Work out the finished part from the listing and answer in its coordinate system (mm). A direction names the side the tool comes from. Round coordinates to 2 decimals unless told otherwise and drop trailing zeros. Order: outer loops, then holes, each group sorted by start corner. A loop starts at its lowest first (then second) coordinate and runs counter-clockwise, first axis right, second up. Notation, with made-up numbers: (-16.5, 56.25) - (-11.5, 56.25) arc R38 cw to (-11.5, 94.25) - close; hole circle Ø3 at (34, 60.25). An arc over 180 degrees is marked (long way). One line per question, with ' | ' between items. Start each with the question number.
from build123d import *

# Parameters (mm, degrees)
F0_R      = 114
F1_DEPTH  = 25
F2_R      = 57
F3_DEPTH  = 200
F4_R      = 114
F5_DEPTH  = 25
F6_R      = 60
F7_DEPTH  = 100
F8_W      = 15
F8_H      = 150
F9_DEPTH  = 25
F10_R     = 9.5
F11_DEPTH = 30
F12_R     = 9.5
F13_DEPTH = 30
F14_R     = 51
F15_DEPTH = 1000


with BuildPart() as f1:
    # F0 (on Front) → F1 (new body)
    with BuildSketch(Plane.XZ):
        Circle(F0_R)
    extrude(amount=F1_DEPTH)

    # F2 (on face) → F3 (join)
    with BuildSketch(Plane.XZ.offset(25)):
        Circle(F2_R)
    extrude(amount=F3_DEPTH)

    # F4 (on face) → F5 (join)
    with BuildSketch(Plane.XZ.offset(225)):
        Circle(F4_R)
    extrude(amount=F5_DEPTH)

    # F6 (on Top) → F7 (join, symmetric)
    with BuildSketch(Plane.XY):
        with Locations((0, -125)):
            Circle(F6_R)
    extrude(amount=F7_DEPTH, both=True)

    # F8 (on face) → F9 (join)
    with BuildSketch(Plane.XY.offset(100)):
        with Locations((-0.883462, -205)):
            Rectangle(F8_W, F8_H)
    extrude(amount=F9_DEPTH)

    # F10 (on face) → F11 (cut)
    with BuildSketch(Plane.XZ.offset(250)):
        with Locations((0, 95)):
            Circle(F10_R)
        with Locations((-67.175144, 67.175144)):
            Circle(F10_R)
        with Locations((-95, 0)):
            Circle(F10_R)
        with Locations((-67.175144, -67.175144)):
            Circle(F10_R)
        with Locations((0, -95)):
            Circle(F10_R)
        with Locations((67.175144, -67.175144)):
            Circle(F10_R)
        with Locations((95, 0)):
            Circle(F10_R)
        with Locations((67.175144, 67.175144)):
            Circle(F10_R)
    extrude(amount=-F11_DEPTH, mode=Mode.SUBTRACT)

    # F12 (on face) → F13 (cut)
    with BuildSketch(Plane(origin=(0, 0, 0), x_dir=(-1, 0, 0), z_dir=(0, 1, 0))):
        with Locations((0, 95)):
            Circle(F12_R)
        with Locations((-67.175144, 67.175144)):
            Circle(F12_R)
        with Locations((-95, 0)):
            Circle(F12_R)
        with Locations((-67.175144, -67.175144)):
            Circle(F12_R)
        with Locations((0, -95)):
            Circle(F12_R)
        with Locations((67.175144, -67.175144)):
            Circle(F12_R)
        with Locations((95, 0)):
            Circle(F12_R)
        with Locations((67.175144, 67.175144)):
            Circle(F12_R)
    extrude(amount=-F13_DEPTH, mode=Mode.SUBTRACT)

    # F14 (on face) → F15 (cut)
    with BuildSketch(Plane(origin=(0, 0, 0), x_dir=(-1, 0, 0), z_dir=(0, 1, 0))):
        Circle(F14_R)
    extrude(amount=-F15_DEPTH, mode=Mode.SUBTRACT)


solid = f1.part
1) Straight lines are drawn through the part: line 1 (Y direction, x = 2, z = 76.5); line 2 (Z direction, x = 0, y = -16.5); line 3 (Z direction, x = 0, y = -234.75). For each, find the intervals that lie inside material, in ascending order.
2) Section D-D on x = 0 is taken. Give the number of separate pieces and of enclosed holes in the cut face, and give its area (3 significant figures).
3) Section B-B on x = -95 is taken. Give the vertices of the cut face in (y, z), and give its area (3 significant figures).
4) For faces 4 (the flat face through (-1, -265, 100)), 5 (the cylindrical face through (58.114, -12.325, -64.322)), 6 (the cylindrical face through (57.23, -106.98, 1.4)), determine the directions among +Z, -Z, +X, -X, +Y, -Y from which every point of the face is accessible in a straight line to the end or side of a thin tool.
5) Determine the mould class of faces 1 (the flat face through (-1, -280, 112)), 2 (the cylindrical face through (-104.061, -12.325, 2.854)), 3 (the cylindrical face through (-12.356, -192.828, -55.645)) for opening direction Y: released by +Y, released by -Y, zero draft, split by the parting line, or undercut.
6) Flat-ended cylindrical pins translate along their axes: pin 1 (8 mm diameter, centred on y = -168.5, z = -68.5, fed in from +X); pin 2 (12 mm diameter, centred on x = -4, y = -210.5, fed in from -Z); pin 3 (10 mm diameter, centred on x = 16.5, y = -129, fed in from -Z); pin 4 (11.5 mm diameter, centred on x = 67.18, z = -67.18, fed in from +Y). Find the tip coordinate at first contact, or state that the pin passes through.
7) Section A-A on y = -125 is taken. Give the vertices of the cut face in (x, z).
8) Section C-C on z = -95 is taken. Give the vertices of the cut face in (x, y).
Recorded:
1) line 1: y = -250 to -225, -184.97 to -65.03, -25 to 0 | line 2: z = -114 to -104.5, -85.5 to -51, 51 to 85.5, 104.5 to 114 | line 3: z = -114 to -104.5, -85.5 to -51, 51 to 85.5, 104.5 to 125
2) separate pieces: 5 | enclosed holes: 0 | area: 20,500 mm²
3) outline: (-250, -63.02) - (-225, -63.02) - (-225, -9.5) - (-250, -9.5) - close; (-250, 9.5) - (-225, 9.5) - (-225, 63.02) - (-250, 63.02) - close; (-25, -63.02) - (0, -63.02) - (0, -9.5) - (-25, -9.5) - close; (-25, 9.5) - (0, 9.5) - (0, 63.02) - (-25, 63.02) - close | area: 5,350 mm²
4) face 4: -Z, +X, -X, -Y | face 5: +Y | face 6: none
5) face 1: released by -Y | face 2: zero draft | face 3: undercut
6) pin 1: stops at x = 45.16 | pin 2: stops at z = -57 | pin 3: stops at z = -100 | pin 4: passes through
7) outline: (-60, -100) - (60, -100) - (60, 100) - (-60, 100) - close; hole circle Ø102 at (0, 0)
8) outline: (-63.02, -250) - (-9.5, -250) - (-9.5, -225) - (-63.02, -225) - close; (-63.02, -25) - (-9.5, -25) - (-9.5, 0) - (-63.02, 0) - close; circle Ø120 at (0, -125); (9.5, -250) - (63.02, -250) - (63.02, -225) - (9.5, -225) - close; (9.5, -25) - (63.02, -25) - (63.02, 0) - (9.5, 0) - close
